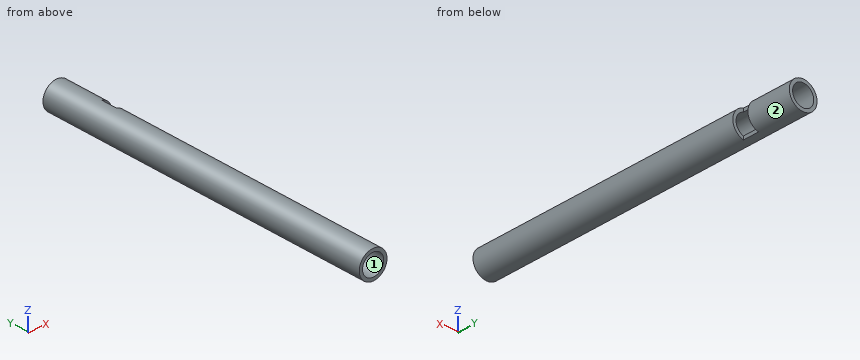
from build123d import *

# Parameters (mm, degrees)
CROQUIS2_R              = 17
CROQUIS2_R_2            = 13
SALIENTE_EXTRUIR1_DEPTH = 420
CROQUIS3_W              = 25
CROQUIS3_H              = 20
CORTAR_EXTRUIR1_DEPTH   = 25


with BuildPart() as part:
    # Croquis2 → Saliente-Extruir1 (new body)
    with BuildSketch(Plane(origin=(0, 0, 0), x_dir=(1, 0, 0), z_dir=(0, 1, 0))):
        Circle(CROQUIS2_R)
        Circle(CROQUIS2_R_2, mode=Mode.SUBTRACT)
    extrude(amount=SALIENTE_EXTRUIR1_DEPTH)

    # Croquis3 → Cortar-Extruir1 (cut, symmetric)
    with BuildSketch(Plane.XY):
        with Locations((16.5, 355)):
            Rectangle(CROQUIS3_W, CROQUIS3_H)
    extrude(amount=CORTAR_EXTRUIR1_DEPTH, both=True, mode=Mode.SUBTRACT)


solid = part.part
Can you work these out from the model? Positions are in its coordinate system, mm. Face numbers are marked on the shaded views. Coordinates: 2 decimals unless noted, no trailing zeros. Order: outer loops, then holes, each group sorted by start corner. A loop starts at its lowest first (then second) coordinate and runs counter-clockwise, first axis right, second up. Notation, with made-up numbers: M 78.25,39 L 93.25,39 A27 ccw 93.25,56 Z; hole C -3,39.5 d8. An arc over 180 degrees is marked long. Answer as CSV lines item,"result".
(1) Suppose I cut it at A-A on z = 0. Please give me the cut outline in (x, y), plus the area to 3 significant figures.
Geometry check:
outline,"M -17,0 L -13,0 L -13,420 L -17,420 Z; M 13,0 L 17,0 L 17,345 L 13,345 Z; M 13,365 L 17,365 L 17,420 L 13,420 Z"
area,"3,280 mm^2"
(2) Suppose I cut it at B-B on x = 0. Please give me the cut outline in (y, z), plus the area to 3 significant figures.
Geometry check:
outline,"M 0,-17 L 420,-17 L 420,-13 L 0,-13 Z; M 0,13 L 420,13 L 420,17 L 0,17 Z"
area,"3,360 mm^2"
(3) Suppose I cut it at C-C on y = 224.5. Please give me the cut outline in (x, z), plus the area to 3 significant figures.
Geometry check:
outline,"C 0,0 d34; hole C 0,0 d26"
area,"377 mm^2"
(4) I'm going to push flat-ended pins straight in: pin 1 (4 mm diameter, centred on y = 102.5, z = -3.5, fed in from -X); pin 2 (12 mm diameter, centred on x = -8.5, y = 217.5, fed in from +Z); pin 3 (1 mm diameter, centred on y = 376, z = 5, fed in from +X). Where does each tip first touch, or does it pass through?
Geometry check:
pin 1,"x = -16.93"
pin 2,"z = 16.82"
pin 3,"x = 16.39"
(5) If we mould it in two halves opening along X, with no side actions, what happens to the marked faces 1 and 2? For each: released by +X, released by -X, zero draft, split by the parting line, or undercut.
Geometry check:
face 1,"undercut"
face 2,"split by the parting line"
(6) Please list where these lines run through material, in increasing order: L1, parallel to X at y = 195, z = 0; L2, parallel to Y at x = 12.5, z = 7; L3, parallel to X at y = 34.5, z = 4.
Geometry check:
L1,"-17 to -13, 13 to 17"
L2,"0 to 345, 365 to 420"
L3,"-16.52 to -12.37, 12.37 to 16.52"
